from build123d import *

# Parameters (mm, degrees)
FLEXTURE_DEPTH                 = 1
GENERAL_START                  = -4.32
GENERAL_DEPTH                  = 4.32
CHANFREIN1_SIZE                = 2
ENL_V_MAT_EXTRU_1_DEPTH        = 2
ESQUISSE2_R                    = 1.75
PASSAGE_VIS_DEPTH              = 54.536972272
LAMAGE_START                   = -1
ESQUISSE2_3_R                  = 2.75
LAMAGE_VIS_DEPTH               = 1.9
ESQUISSE3_R                    = 2.75
IMPRESSIONBRIDGE_DEPTH         = 0.4
SYM_TRIE_2_VIS_COPY_1_SKETCH_R = 1.75
SYM_TRIE_2_VIS_COPY_1_DEPTH    = 54.536972272
SYM_TRIE_START                 = -1
SYM_TRIE_2_VIS_COPY_2_SKETCH_R = 2.75
SYM_TRIE_2_VIS_COPY_2_DEPTH    = 1.9
SYM_TRIE_2_VIS_COPY_3_SKETCH_R = 2.75
SYM_TRIE_2_VIS_COPY_3_DEPTH    = 0.4


with BuildPart() as part:
    # Esquisse1 → Flexture (new body)
    with BuildSketch(Plane.XY):
        with BuildLine():
            ThreePointArc((40.15, 20.15), (35.756601718, 30.756601718), (25.15, 35.15))
            Line((25.15, 35.15), (-25.15, 35.15))
            ThreePointArc((-25.15, 35.15), (-35.756601718, 30.756601718), (-40.15, 20.15))
            Line((-40.15, 20.15), (-40.15, -20.15))
            ThreePointArc((-40.15, -20.15), (-35.756601718, -30.756601718), (-25.15, -35.15))
            Line((-25.15, -35.15), (25.15, -35.15))
            ThreePointArc((25.15, -35.15), (35.756601718, -30.756601718), (40.15, -20.15))
            Line((40.15, -20.15), (40.15, 20.15))
        make_face()
        with BuildLine():
            Line((9.944420337, 6.246632211), (9.024077951, 6.246632211))
            ThreePointArc((9.024077951, 6.246632211), (7.609864388, 6.832418648), (7.024077951, 8.246632211))
            Line((7.024077951, 8.246632211), (7.024077951, 11.421689431))
            ThreePointArc((7.024077951, 11.421689431), (8.90907126, 13.478916909), (11.122855622, 11.780522528))
            ThreePointArc((11.122855622, 11.780522528), (11.128556545, 11.737248439), (11.130461693, 11.693642044))
            ThreePointArc((11.130461693, 11.693642044), (23.380482865, 6.619517135), (18.306357956, 18.869538307))
            ThreePointArc((18.306357956, 18.869538307), (17.806357956, 19.369538307), (18.306357956, 19.869538307))
            ThreePointArc((18.306357956, 19.869538307), (26.07883242, 9.157124665), (13.483641052, 5.091621037))
            ThreePointArc((13.483641052, 5.091621037), (11.805880388, 5.950575275), (9.944420337, 6.246632211))
        make_face(mode=Mode.SUBTRACT)
        with BuildLine():
            ThreePointArc((-18.306357956, -18.869538307), (-17.806357956, -19.369538307), (-18.306357956, -19.869538307))
            ThreePointArc((-18.306357956, -19.869538307), (-24.087589646, -5.912410354), (-10.130461693, -11.693642044))
            ThreePointArc((-10.130461693, -11.693642044), (-10.630461693, -12.193642044), (-11.130461693, -11.693642044))
            ThreePointArc((-11.130461693, -11.693642044), (-23.380482865, -6.619517135), (-18.306357956, -18.869538307))
        make_face(mode=Mode.SUBTRACT)
        with BuildLine():
            ThreePointArc((11.130461693, -11.693642044), (10.630461693, -12.193642044), (10.130461693, -11.693642044))
            ThreePointArc((10.130461693, -11.693642044), (24.087589646, -5.912410354), (18.306357956, -19.869538307))
            ThreePointArc((18.306357956, -19.869538307), (17.806357956, -19.369538307), (18.306357956, -18.869538307))
            ThreePointArc((18.306357956, -18.869538307), (23.380482865, -6.619517135), (11.130461693, -11.693642044))
        make_face(mode=Mode.SUBTRACT)
        with BuildLine():
            ThreePointArc((-18.306357956, 18.869538307), (-23.380482865, 6.619517135), (-11.130461693, 11.693642044))
            ThreePointArc((-11.130461693, 11.693642044), (-10.630461693, 12.193642044), (-10.130461693, 11.693642044))
            ThreePointArc((-10.130461693, 11.693642044), (-24.087589646, 5.912410354), (-18.306357956, 19.869538307))
            ThreePointArc((-18.306357956, 19.869538307), (-17.806357956, 19.369538307), (-18.306357956, 18.869538307))
        make_face(mode=Mode.SUBTRACT)
    extrude(amount=FLEXTURE_DEPTH)

    # Esquisse1<6> → General (add)
    with BuildSketch(Plane.XY.offset(GENERAL_START)):
        with BuildLine():
            Line((25.15, 35.15), (-25.15, 35.15))
            ThreePointArc((-25.15, 35.15), (-35.756601718, 30.756601718), (-40.15, 20.15))
            Line((-40.15, 20.15), (-40.15, -20.15))
            ThreePointArc((-40.15, -20.15), (-35.756601718, -30.756601718), (-25.15, -35.15))
            Line((-25.15, -35.15), (25.15, -35.15))
            ThreePointArc((25.15, -35.15), (35.756601718, -30.756601718), (40.15, -20.15))
            Line((40.15, -20.15), (40.15, 20.15))
            ThreePointArc((40.15, 20.15), (35.756601718, 30.756601718), (25.15, 35.15))
        make_face()
        with BuildLine():
            Line((-27.65, 20.15), (-27.65, -20.15))
            ThreePointArc((-27.65, -20.15), (-26.917766953, -21.917766953), (-25.15, -22.65))
            Line((-25.15, -22.65), (25.15, -22.65))
            ThreePointArc((25.15, -22.65), (26.917766953, -21.917766953), (27.65, -20.15))
            Line((27.65, -20.15), (27.65, 20.15))
            ThreePointArc((27.65, 20.15), (26.917766953, 21.917766953), (25.15, 22.65))
            Line((25.15, 22.65), (-25.15, 22.65))
            ThreePointArc((-25.15, 22.65), (-26.917766953, 21.917766953), (-27.65, 20.15))
        make_face(mode=Mode.SUBTRACT)
    extrude(amount=GENERAL_DEPTH)

    # Chanfrein1
    chanfrein1_edges = [part.edges().sort_by_distance(p)[0] for p in [
        (35.756601718, 30.756601718, 1),
        (0, 35.15, 1),
        (-35.756601718, 30.756601718, 1),
        (-40.15, 0, 1),
        (-35.756601718, -30.756601718, 1),
        (0, -35.15, 1),
        (35.756601718, -30.756601718, 1),
        (40.15, 0, 1),
    ]]
    chamfer(chanfrein1_edges, length=CHANFREIN1_SIZE)

    # Esquisse4 → Enlèv. mat.-Extru.1 (cut)
    with BuildSketch(Plane(origin=(0, 0, -4.32), x_dir=(-1, 0, 0), z_dir=(0, 0, -1))):
        with BuildLine():
            Line((-40.15, -20.15), (-40.15, 20.15))
            ThreePointArc((-40.15, 20.15), (-35.756601718, 30.756601718), (-25.15, 35.15))
            Line((-25.15, 35.15), (25.15, 35.15))
            ThreePointArc((25.15, 35.15), (35.756601718, 30.756601718), (40.15, 20.15))
            Line((40.15, 20.15), (40.15, -20.15))
            ThreePointArc((40.15, -20.15), (35.756601718, -30.756601718), (25.15, -35.15))
            Line((25.15, -35.15), (-25.15, -35.15))
            ThreePointArc((-25.15, -35.15), (-35.756601718, -30.756601718), (-40.15, -20.15))
        make_face()
        with BuildLine():
            Line((25.15, -33.65), (-25.15, -33.65))
            ThreePointArc((-25.15, -33.65), (-34.695941546, -29.695941546), (-38.65, -20.15))
            Line((-38.65, -20.15), (-38.65, 20.15))
            ThreePointArc((-38.65, 20.15), (-34.695941546, 29.695941546), (-25.15, 33.65))
            Line((-25.15, 33.65), (25.15, 33.65))
            ThreePointArc((25.15, 33.65), (34.695941546, 29.695941546), (38.65, 20.15))
            Line((38.65, 20.15), (38.65, -20.15))
            ThreePointArc((38.65, -20.15), (34.695941546, -29.695941546), (25.15, -33.65))
        make_face(mode=Mode.SUBTRACT)
    extrude(amount=-ENL_V_MAT_EXTRU_1_DEPTH, mode=Mode.SUBTRACT)

    # Esquisse2 → Passage vis (cut, through all)
    with BuildSketch(Plane(origin=(0, 0, 0), x_dir=(-1, 0, 0), z_dir=(0, 0, -1))):
        with Locations((-30.276524164, 25.276524164)):
            Circle(ESQUISSE2_R)
    passage_vis = extrude(amount=PASSAGE_VIS_DEPTH, mode=Mode.SUBTRACT)

    # Esquisse2<3> → Lamage vis (cut)
    with BuildSketch(Plane(origin=(0, 0, 0), x_dir=(-1, 0, 0), z_dir=(0, 0, -1)).offset(LAMAGE_START)):
        with Locations(Location((-30.276524164, 25.276524164, 0), (0, 0, 180))):
            Circle(ESQUISSE2_3_R)
    lamage_vis = extrude(amount=LAMAGE_VIS_DEPTH, mode=Mode.SUBTRACT)

    # Esquisse3 → ImpressionBridge (add)
    with BuildSketch(Plane.XY.offset(-0.9)):
        with Locations((30.276524164, 25.276524164)):
            Circle(ESQUISSE3_R)
    impressionbridge = extrude(amount=-IMPRESSIONBRIDGE_DEPTH)

    # Symétrie vis: Passage vis, Lamage vis, ImpressionBridge across plane
    add(passage_vis.mirror(Plane(origin=(0, 0, 0), x_dir=(0, 0, 1), z_dir=(1, 0, 0))), mode=Mode.SUBTRACT)
    add(lamage_vis.mirror(Plane(origin=(0, 0, 0), x_dir=(0, 0, 1), z_dir=(1, 0, 0))), mode=Mode.SUBTRACT)
    add(impressionbridge.mirror(Plane(origin=(0, 0, 0), x_dir=(0, 0, 1), z_dir=(1, 0, 0))))

    # Symétrie 2 vis: Passage vis, Lamage vis, ImpressionBridge across plane
    add(passage_vis.mirror(Plane.ZX), mode=Mode.SUBTRACT)
    add(lamage_vis.mirror(Plane.ZX), mode=Mode.SUBTRACT)
    add(impressionbridge.mirror(Plane.ZX))

    # Symétrie 2 vis copy 1 sketch → Symétrie 2 vis copy 1 (cut, through all)
    with BuildSketch(Plane(origin=(0, 0, 0), x_dir=(1, 0, 0), z_dir=(0, 0, -1))):
        with Locations((-30.276524164, 25.276524164)):
            Circle(SYM_TRIE_2_VIS_COPY_1_SKETCH_R)
    extrude(amount=SYM_TRIE_2_VIS_COPY_1_DEPTH, mode=Mode.SUBTRACT)

    # Symétrie 2 vis copy 2 sketch → Symétrie 2 vis copy 2 (cut)
    with BuildSketch(Plane(origin=(0, 0, 0), x_dir=(1, 0, 0), z_dir=(0, 0, -1)).offset(SYM_TRIE_START)):
        with Locations(Location((-30.276524164, 25.276524164, 0), (0, 0, 180))):
            Circle(SYM_TRIE_2_VIS_COPY_2_SKETCH_R)
    extrude(amount=SYM_TRIE_2_VIS_COPY_2_DEPTH, mode=Mode.SUBTRACT)

    # Symétrie 2 vis copy 3 sketch → Symétrie 2 vis copy 3 (add)
    with BuildSketch(Plane(origin=(0, 0, -0.9), x_dir=(-1, 0, 0), z_dir=(0, 0, 1))):
        with Locations((30.276524164, 25.276524164)):
            Circle(SYM_TRIE_2_VIS_COPY_3_SKETCH_R)
    extrude(amount=-SYM_TRIE_2_VIS_COPY_3_DEPTH)


solid = part.part
Build history of the part. All positions in model axes, mm. A direction names the side the tool comes from. Coordinates: 2 decimals unless noted, no trailing zeros. Order: outer loops, then holes, each group sorted by start corner. A loop starts at its lowest first (then second) coordinate and runs counter-clockwise, first axis right, second up. Notation, with made-up numbers: (75, 45) - (129, 45) arc R16 ccw to (129, 68) - close; hole circle Ø4 at (45, -7.75). An arc over 180 degrees is marked (long way). Write item = value, one per line. Start each with the question number.
1) Two-plate mould, pull along X, no slides. Class faces 1 (the face through (23.89, -5.72, 0.49)), 2 (the face through (-1, 0, 1)), 3 (the face through (-34.8, -29.59, -3.33)): pulls with the +X half, pulls with the -X half, needs draft (parallel to the pull), parting line crosses it, or undercut.
2) 3-axis set-ups, long thin cutter, end or side, ignore diameter. For faces 4 (the face through (0, 33.65, -3)), 5 (the face through (-30, -25, -0.9)), 6 (the face through (30, 25, -1.3)), 7 (the face through (-34.59, 29.8, -3.33)): which of +Z, -Z, +X, -X, +Y, -Y reach the whole face in a straight line?
3) Saw through at C-C on x = 4. Write the cut outline in (y, z).
4) Wall check: line 1 along Y through (x, z) = (-14.5, -3.1); line 2 along X through (y, z) = (4, -4.1). Give the ranges that are in metal, low to high. Write a range as from..to.
5) Saw through at D-D on y = -18. Write the cut outline in (x, z).
6) Flat gauge pins, fed straight in: pin 1 Ø2 at (y, z) = (-11, -3.5) entering from -X; pin 2 Ø9 at (x, y) = (30.28, -25.28) entering from -Z; pin 3 Ø1 at (x, y) = (29.5, 25) entering from -Z; pin 4 Ø10 at (x, y) = (-7.5, 16) entering from -Z. Where does each tip first touch, or does it go through?
7) Saw through at A-A on x = 22.5. Count the separate pieces of the cut face and the enclosed holes in it, then the cut area to 3 significant figures.
From the geometry:
q1.face_1 = undercut
q1.face_2 = needs draft
q1.face_3 = pulls with the -X half
q2.face_4 = -Z, +X, -X, +Y
q2.face_5 = +Z
q2.face_6 = -Z
q2.face_7 = -Z, -X, +Y
q3.outline = (-35.15, -2.32) - (-33.65, -2.32) - (-33.65, -4.32) - (-22.65, -4.32) - (-22.65, 0) - (22.65, 0) - (22.65, -4.32) - (33.65, -4.32) - (33.65, -2.32) - (35.15, -2.32) - (35.15, -1) - (33.15, 1) - (-33.15, 1) - (-35.15, -1) - close
q4.line_1 = -33.65..-22.65, 22.65..33.65
q4.line_2 = -38.65..-27.65, 27.65..38.65
q5.outline = (-40.15, -2.32) - (-38.65, -2.32) - (-38.65, -4.32) - (-27.65, -4.32) - (-27.65, 0) - (-23.51, 0) - (-23.51, 1) - (-38.15, 1) - (-40.15, -1) - close; (-21.73, 0) - (21.73, 0) - (21.73, 1) - (-21.73, 1) - close; (23.51, 0) - (27.65, 0) - (27.65, -4.32) - (38.65, -4.32) - (38.65, -2.32) - (40.15, -2.32) - (40.15, -1) - (38.15, 1) - (23.51, 1) - close
q6.pin_1 = -38.65
q6.pin_2 = -4.32
q6.pin_3 = -1.3
q6.pin_4 = 0
q7.separate_pieces = 5
q7.enclosed_holes = 0
q7.area = 164 mm^2
